Geometry check sheet. Reference: the model listing, model coordinates, mm. Face numbers are marked on the shaded views. Round coordinates to 2 decimals unless told otherwise and drop trailing zeros. Loops run counter-clockwise (first coordinate to the right, second up) from the corner with the lowest first, then second, coordinate; pieces in that order, holes last. Notation, with made-up numbers: (32, 76.25) -> (46, 76.25) arc R34 cw to (46, 106.25) -> close; hole circle Ø4 at (86.5, 7.25). An arc over 180 degrees is marked (long way). Use a Markdown table: item, result. Add a question column.
Q1. Material ranges on L1, parallel to Y at x = 6, z = 0.05; L2, parallel to X at y = -2, z = -0.8; L3, parallel to X at y = 0.55, z = -1.6, recorded low to high.
Q2. Sectioned sample at A-A, the plane z = 0. Enter the section's corners in (x, y), then the cut area to 3 significant figures.
Q3. Sectioned sample at D-D, the plane x = 2. Enter the section's corners in (y, z), then the cut area to 3 significant figures.
Q4. Sectioned sample at B-B, the plane y = 0. Enter the section's corners in (x, z), then the cut area to 3 significant figures.
Q5. Gauge pin test, flat ends, axial feed: P1, Ø0.6, axis at x = 0.5, z = -0.5, coming from the -Y side; P2, Ø0.6, axis at x = 0.5, z = 0.5, coming from the +Y side. Record the tip position at first contact, or that the pin passes through.
Q6. Sectioned sample at C-C, the plane x = 1. Enter the section's corners in (y, z), then the cut area to 3 significant figures.
Q7. Release check for a two-part mould opening along Y. For the marked faces 1, 2 and 3 record: released by +Y, released by -Y, zero draft, split by the parting line, or undercut.
```python
from build123d import *

# Parameters (mm, degrees)
ZKOSIT1_SIZE             = 0.21
ZAOBLIT1_R               = 0.1
SKICA3_W                 = 5
SKICA3_H                 = 0.8
ODEBRAT_VYSUNUT_M2_DEPTH = 1.2


with BuildPart() as part:
    # Skica1 → Otočit kolem osy1 (revolve)
    with BuildSketch(Plane(origin=(0, 0, 0), x_dir=(1, 0, 0), z_dir=(0, 1, 0))):
        with BuildLine():
            Line((2.5, 2.5), (2.5, 1.5))
            Line((2.5, 1.5), (8.5, 1.5))
            Line((8.5, 1.5), (8.5, 0))
            Line((8.5, 0), (0, 0))
            ThreePointArc((0, 0), (0.732233047, 1.767766953), (2.5, 2.5))
        make_face()
    revolve(axis=Axis((0, 0, 0), (1, 0, 0)))

    # Zkosit1
    zkosit1_edges = [part.edges().sort_by_distance(p)[0] for p in [
        (8.5, 0, 1.5),
    ]]
    chamfer(zkosit1_edges, length=ZKOSIT1_SIZE)

    # Zaoblit1
    zaoblit1_edges = [part.edges().sort_by_distance(p)[0] for p in [
        (2.5, 0, 1.5),
    ]]
    fillet(zaoblit1_edges, radius=ZAOBLIT1_R)

    # Skica3 → Odebrat vysunutím2 (cut)
    with BuildSketch(Plane(origin=(0, 0, 0), x_dir=(0, 0, -1), z_dir=(1, 0, 0))):
        Rectangle(SKICA3_W, SKICA3_H)
    extrude(amount=ODEBRAT_VYSUNUT_M2_DEPTH, mode=Mode.SUBTRACT)


solid = part.part
```
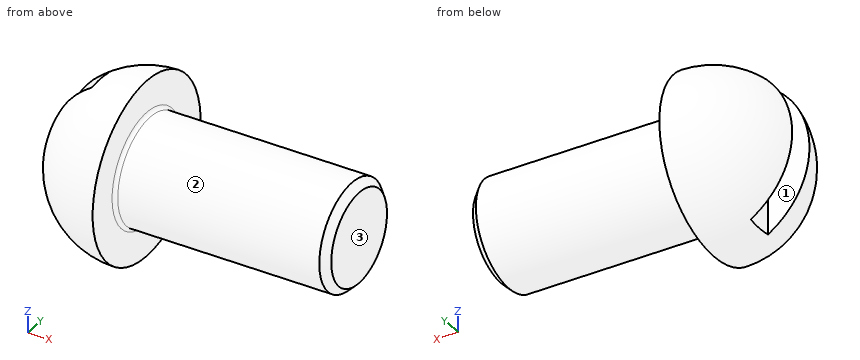
Values:
| question | item | result |
|---|---|---|
| 1 | L1 | -1.5 to 1.5 |
| 1 | L2 | 1.23 to 2.5 |
| 1 | L3 | 0.66 to 2.5 |
| 2 | outline | (0.03, -0.4) arc R2.5 ccw to (2.5, -2.5) -> (2.5, -1.6) arc R0.1 cw to (2.6, -1.5) -> (8.29, -1.5) -> (8.5, -1.29) -> (8.5, 1.29) -> (8.29, 1.5) -> (2.6, 1.5) arc R0.1 cw to (2.5, 1.6) -> (2.5, 2.5) arc R2.5 ccw to (0.03, 0.4) -> (1.2, 0.4) -> (1.2, -0.4) -> close |
| 2 | area | 26.8 mm^2 |
| 3 | outline | circle Ø4.9 at (0, 0) |
| 3 | area | 18.8 mm^2 |
| 4 | outline | (1.2, -2.14) arc R2.5 ccw to (2.5, -2.5) -> (2.5, -1.6) arc R0.1 cw to (2.6, -1.5) -> (8.29, -1.5) -> (8.5, -1.29) -> (8.5, 1.29) -> (8.29, 1.5) -> (2.6, 1.5) arc R0.1 cw to (2.5, 1.6) -> (2.5, 2.5) arc R2.5 ccw to (1.2, 2.14) -> close |
| 4 | area | 24.2 mm^2 |
| 5 | P1 | y = -1.77 |
| 5 | P2 | y = 1.77 |
| 6 | outline | (-0.4, -1.96) -> (-0.4, 1.96) arc R2 ccw to start; (0.4, -1.96) arc R2 ccw to (0.4, 1.96) -> close |
| 6 | area | 9.39 mm^2 |
| 7 | face 1 | undercut |
| 7 | face 2 | split by the parting line |
| 7 | face 3 | zero draft |
